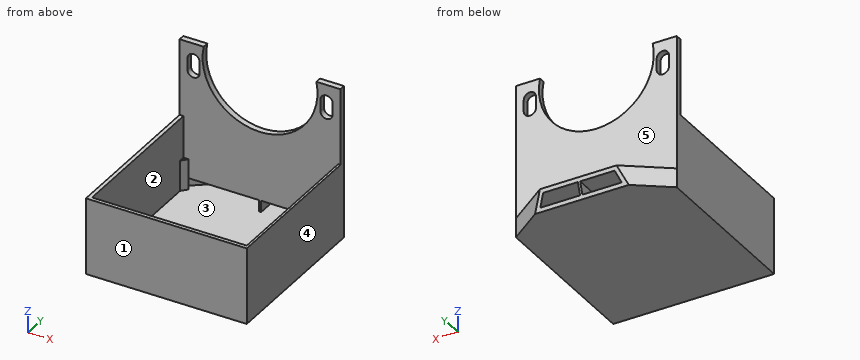
from build123d import *

# Parameters (mm, degrees)
SKETCH_1_W               = 42
SKETCH_1_H               = 43
EXTRUDE_1_DEPTH          = 20
SKETCH_2_W               = 40.4
SKETCH_2_H               = 40.4
CUT_EXTRUDE_1_DEPTH      = 19
EXTRUDE_2_DEPTH          = 5
CUT_EXTRUDE_2_DEPTH      = 3
EXTRUDE_3_DEPTH          = 8
SKETCH_7_W               = 42
SKETCH_7_H               = 1.6
EXTRUDE_4_DEPTH          = 20
SKETCH_8_R               = 15
CUT_EXTRUDE_3_DEPTH      = 20
SKETCH_9_W               = 0.6
SKETCH_9_H               = 9.6
EXTRUDE_5_DEPTH          = 3
CUT_EXTRUDE_4_DEPTH      = 20
CUT_EXTRUDE_4_DEPTH_BACK = 20


with BuildPart() as part:
    # 草图1 → 凸台-拉伸1 (new body)
    with BuildSketch(Plane.XY):
        with Locations((21, 21.5)):
            Rectangle(SKETCH_1_W, SKETCH_1_H)
    extrude(amount=EXTRUDE_1_DEPTH)

    # 草图2 → 切除-拉伸1 (cut)
    with BuildSketch(Plane.XY.offset(20)):
        with Locations((21.2, 21.2)):
            Rectangle(SKETCH_2_W, SKETCH_2_H)
    extrude(amount=-CUT_EXTRUDE_1_DEPTH, mode=Mode.SUBTRACT)

    # 草图3 → 凸台-拉伸2 (add)
    with BuildSketch(Plane(origin=(0, 0, 0), x_dir=(-1, 0, 0), z_dir=(0, 0, -1))):
        Polygon((-42, 43), (0, 43), (-11, 51), (-31, 51), align=None)
    extrude(amount=-EXTRUDE_2_DEPTH)

    # 草图5 → 切除-拉伸2 (cut)
    with BuildSketch(Plane.XY.offset(1)):
        Polygon((1, 41.4), (1, 42.434468933), (13.156473194, 51.802822617), (28.849580276, 51.802822617), (41.4, 42.434468933), (41.4, 41.4), align=None)
    extrude(amount=CUT_EXTRUDE_2_DEPTH, mode=Mode.SUBTRACT)

    # 草图6 → 凸台-拉伸3 (add)
    with BuildSketch(Plane.XY.offset(1)):
        Polygon((1, 41.4), (1, 39.954103811), (2.344864369, 41.4), align=None)
        Polygon((41.4, 41.4), (41.4, 39.954103811), (39.954103811, 41.4), align=None)
        Polygon((41.4, 1), (41.4, 2.836916903), (39.563083097, 1), align=None)
        Polygon((1, 1), (1, 2.836916903), (2.836916903, 1), align=None)
    extrude(amount=EXTRUDE_3_DEPTH)

    # 草图7 → 凸台-拉伸4 (add)
    with BuildSketch(Plane.XY.offset(20)):
        with Locations((21, 42.2)):
            Rectangle(SKETCH_7_W, SKETCH_7_H)
    extrude(amount=EXTRUDE_4_DEPTH)

    # 草图8 → 切除-拉伸3 (cut)
    with BuildSketch(Plane.XZ.offset(-41.4)):
        with Locations((21, 37.088393363)):
            Circle(SKETCH_8_R)
        with BuildLine():
            Line((2.04, 32.61), (2.04, 35.61))
            ThreePointArc((2.04, 35.61), (3.64, 37.21), (5.24, 35.61))
            Line((5.24, 35.61), (5.24, 32.61))
            ThreePointArc((5.24, 32.61), (3.64, 31.01), (2.04, 32.61))
        make_face()
        with BuildLine():
            Line((39.96, 32.61), (39.96, 35.61))
            ThreePointArc((39.96, 35.61), (38.36, 37.21), (36.76, 35.61))
            Line((36.76, 35.61), (36.76, 32.61))
            ThreePointArc((36.76, 32.61), (38.36, 31.01), (39.96, 32.61))
        make_face()
    extrude(amount=-CUT_EXTRUDE_3_DEPTH, mode=Mode.SUBTRACT)

    # 草图9 → 凸台-拉伸5 (add)
    with BuildSketch(Plane.XY.offset(1)):
        with Locations((21, 46.2)):
            Rectangle(SKETCH_9_W, SKETCH_9_H)
    extrude(amount=EXTRUDE_5_DEPTH)

    # 草图10 → 切除-拉伸4 (cut, two sides: drawn at the far end of the back side and taken through both)
    with BuildSketch(Plane.ZY.offset(-20.7).offset(-CUT_EXTRUDE_4_DEPTH_BACK)):
        Polygon((5, 51), (-3.034223026, 48.389522695), (-3.034223026, 51), align=None)
    extrude(amount=CUT_EXTRUDE_4_DEPTH + CUT_EXTRUDE_4_DEPTH_BACK, mode=Mode.SUBTRACT)


solid = part.part
Input: part model. Units: mm. Frame: model coordinates. Face numbers are marked on the shaded views. A direction names the side the tool comes from. Coordinates: 2 decimals unless noted, no trailing zeros. Order: outer loops, then holes, each group sorted by start corner. A loop starts at its lowest first (then second) coordinate and runs counter-clockwise, first axis right, second up. Notation, with made-up numbers: M 68,60 L 74,60 A16 cw 74,65 Z; hole C -30.5,38 d11. An arc over 180 degrees is marked long. Answer as CSV lines item,"result".
1. Section D-D (y = 13). Return the cut outline in (x, z).
Reported:
outline,"M 0,0 L 42,0 L 42,20 L 41.4,20 L 41.4,1 L 1,1 L 1,20 L 0,20 Z"
2. Material intervals for line 1 (X direction, y = 4, z = 8); line 2 (Y direction, x = 3, z = 14); line 3 (Z direction, x = 32, y = 16.5), sorted ascending. Write a range as from..to.
Reported:
line 1,"0..1, 41.4..42"
line 2,"0..1, 41.4..43"
line 3,"0..1"
3. Access query for the marked faces 1 and 2. Directions: +Z, -Z, +X, -X, +Y, -Y. A direction counts if a zero-diameter tool reaches every point of the face in a straight line with its end or side. Return the directions, or none.
Reported:
face 1,"+Z, -Z, +X, -X, -Y"
face 2,"+Z"
4. Section A-A (z = 15). Return the cut outline in (x, y).
Reported:
outline,"M 0,0 L 42,0 L 42,43 L 0,43 Z; hole M 1,1 L 41.4,1 L 41.4,41.4 L 1,41.4 Z"
5. Section B-B (x = 14). Return the cut outline in (y, z).
Reported:
outline,"M 0,0 L 49.38,0 L 49.7,1 L 1,1 L 1,20 L 0,20 Z; M 41.4,4 L 50.68,4 L 51,5 L 43,5 L 43,23.82 L 41.4,23.82 Z"
6. Section C-C (y = 48). Return the cut outline in (x, z) (3 decimals), then the cut area to 3 significant figures.
Reported:
outline,"M 6.875,0 L 35.125,0 L 35.125,5 L 6.875,5 Z; hole M 8.222,1 L 20.7,1 L 20.7,4 L 8.222,4 Z; hole M 21.3,1 L 33.944,1 L 33.944,4 L 21.3,4 Z"
area,"65.9 mm2"
7. Pull-direction query (Y, two-part tool) for the marked faces 3, 4 and 5; classes: released by +Y, released by -Y, zero draft, split by the parting line, or undercut.
Reported:
face 3,"undercut"
face 4,"zero draft"
face 5,"released by +Y"
8. First-contact query: P1, Ø12, axis at x = 34.5, z = 23, coming from the +Y side; P2, Ø12.5, axis at x = 13, y = 25.5, coming from the +Z side; P3, Ø2, axis at x = 2, y = 1.5, coming from the +Z side. Flat tips, straight axial feed; report the tip coordinate or a pass-through.
Reported:
P1,"y = 43"
P2,"z = 1"
P3,"z = 20"
